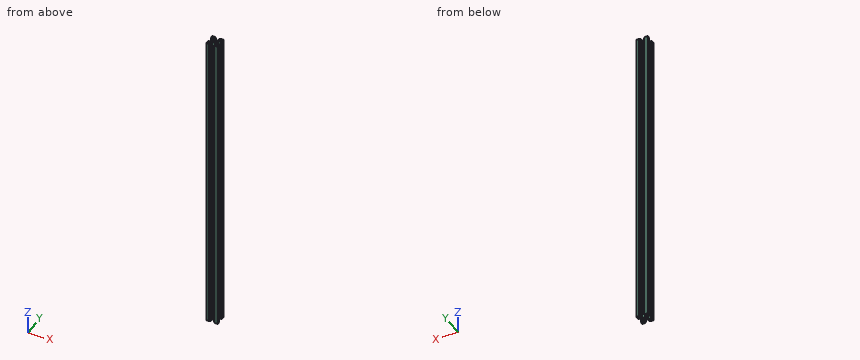
from build123d import *

# Parameters (mm, degrees)
F1_DEPTH = 550
F2_R     = 2.1
F3_DEPTH = 550.001


with BuildPart() as f1:
    # F0 (on Top) → F1 (new body)
    with BuildSketch(Plane.XY):
        Polygon((0, 5.2), (0, 0), (5.2, 0), (7, 1.8), (4.4, 1.8), (4.4, 3.44), (7.16, 6.2), (12.84, 6.2), (15.6, 3.44), (15.6, 1.8), (13, 1.8), (14.8, 0), (20, 0), (20, 5.2), (18.2, 7), (18.2, 4.4), (16.56, 4.4), (13.8, 7.16), (13.8, 12.84), (16.56, 15.6), (18.2, 15.6), (18.2, 13), (20, 14.8), (20, 20), (14.8, 20), (13, 18.2), (15.6, 18.2), (15.6, 16.56), (12.84, 13.8), (7.16, 13.8), (4.4, 16.56), (4.4, 18.2), (7, 18.2), (5.2, 20), (0, 20), (0, 14.8), (1.8, 13), (1.8, 15.6), (3.44, 15.6), (6.2, 12.84), (6.2, 7.16), (3.44, 4.4), (1.8, 4.4), (1.8, 7), align=None)
    extrude(amount=F1_DEPTH)

    # F2 (on face) → F3 (cut, through all)
    with BuildSketch(Plane.XY.offset(550)):
        with Locations((10, 10)):
            Circle(F2_R)
        Polygon((18.2, 16.67), (18.2, 18.2), (16.67, 18.2), align=None)
        Polygon((3.33, 18.2), (1.8, 18.2), (1.8, 16.67), align=None)
        Polygon((1.8, 3.33), (1.8, 1.8), (3.33, 1.8), align=None)
        Polygon((16.67, 1.8), (18.2, 1.8), (18.2, 3.33), align=None)
    extrude(amount=-F3_DEPTH, mode=Mode.SUBTRACT)


solid = f1.part
Model file for the job. Use its own axes, mm. Give positions to 0.01 mm unless a question says otherwise; leave off trailing zeros. Answer as CSV lines item,"result".
1. Drill centre lines: L1, parallel to Y at x = 10, z = 345.5; L2, parallel to Y at x = 17.5, z = 291; L3, parallel to Y at x = 6.5, z = 61.5. Where is each one in solid material? Low to high. Write a range as [from, to].
Responses:
L1,"y = [6.2, 7.9], [12.1, 13.8]"
L2,"y = [0, 1.8], [2.63, 4.4], [15.6, 17.37], [18.2, 20]"
L3,"y = [1.3, 1.8], [5.54, 14.46], [18.2, 18.7]"
2. Band-saw the part on A-A (z = 486). Count the separate pieces of the cut face and the enclosed holes in it, and give its area (3 significant figures).
Responses:
separate pieces,"1"
enclosed holes,"5"
area,"159 mm2"
3. Pin check, flat tips, straight feed: pin 1 (1.3 mm diameter, centred on y = 6, z = 271.5, fed in from -X); pin 2 (6 mm diameter, centred on y = 8.5, z = 141, fed in from +X); pin 3 (4.5 mm diameter, centred on x = 9.5, z = 380, fed in from +Y). Stop position of each tip, or through.
Responses:
pin 1,"stops at x = 0.15"
pin 2,"stops at x = 19.7"
pin 3,"stops at y = 13.8"
